from build123d import *

# Parameters (mm, degrees)
SKETCH2_W               = 100
SKETCH2_H               = 65
BOSS_EXTRUDE1_DEPTH     = 25
SKETCH3_W               = 40
SKETCH3_H               = 65
BOSS_EXTRUDE2_DEPTH     = 50
SKETCH4_W               = 50
SKETCH4_H               = 20
CUT_EXTRUDE1_DEPTH      = 40
CUT_EXTRUDE2_DEPTH      = 139.406105357
CUT_EXTRUDE2_DEPTH_BACK = 139.406105357
SKETCH5_W               = 41
SKETCH5_H               = 5.985076192
CUT_EXTRUDE4_START      = -25
SKETCH6_W               = 40
SKETCH6_H               = 25
CUT_EXTRUDE4_DEPTH      = 25


with BuildPart() as part:
    # Sketch2 → Boss-Extrude1 (new body)
    with BuildSketch(Plane(origin=(0, 0, 0), x_dir=(1, 0, 0), z_dir=(0, 1, 0))):
        Rectangle(SKETCH2_W, SKETCH2_H)
    extrude(amount=BOSS_EXTRUDE1_DEPTH)

    # Sketch3 → Boss-Extrude2 (add, symmetric)
    with BuildSketch(Plane(origin=(0, 0, 0), x_dir=(0, 0, -1), z_dir=(1, 0, 0))):
        with Locations((12.5, 57.5)):
            Rectangle(SKETCH3_W, SKETCH3_H)
    extrude(amount=BOSS_EXTRUDE2_DEPTH, both=True)

    # Sketch4 → Cut-Extrude1 (cut)
    with BuildSketch(Plane(origin=(0, 90, 0), x_dir=(1, 0, 0), z_dir=(0, 1, 0))):
        with Locations((0, 2.5)):
            Rectangle(SKETCH4_W, SKETCH4_H)
    extrude(amount=-CUT_EXTRUDE1_DEPTH, mode=Mode.SUBTRACT)

    # Sketch5 → Cut-Extrude2 (cut, two sides: drawn at the far end of the back side and taken through both)
    with BuildSketch(Plane(origin=(50, 0, 0), x_dir=(0, 0, -1), z_dir=(1, 0, 0)).offset(-CUT_EXTRUDE2_DEPTH_BACK)):
        with Locations((0, 2.992538096)):
            Rectangle(SKETCH5_W, SKETCH5_H)
    extrude(amount=CUT_EXTRUDE2_DEPTH + CUT_EXTRUDE2_DEPTH_BACK, mode=Mode.SUBTRACT)

    # Sketch6 → Cut-Extrude4 (cut)
    with BuildSketch(Plane.XY.offset(32.5).offset(CUT_EXTRUDE4_START)):
        with Locations((0, 12.5)):
            Rectangle(SKETCH6_W, SKETCH6_H)
    extrude(amount=CUT_EXTRUDE4_DEPTH, mode=Mode.SUBTRACT)


solid = part.part
Input: part model. Units: mm. Frame: model coordinates. A direction names the side the tool comes from. Round coordinates to 2 decimals unless told otherwise and drop trailing zeros. Order: outer loops, then holes, each group sorted by start corner. A loop starts at its lowest first (then second) coordinate and runs counter-clockwise, first axis right, second up. Notation, with made-up numbers: (26.5, 73.5) - (43.5, 73.5) arc R30 ccw to (43.5, 95.5) - close; hole circle Ø5 at (45.5, 36.25). An arc over 180 degrees is marked (long way). Answer as a JSON object with one key per item and string values. Group by question number.
(1) Reachability of faces 5 (the face through (-35, 25, 20)), 6 (the face through (-1, 5.985, 0)), 7 (the face through (20, 12, 20)) from +Z, -Z, +X, -X, +Y, -Y: full face, straight path, thin tool, end or side. Return the list, or none.
(2) Cut plane C-C (x = 29). Return loops of the section in (y, z).
(3) Draft query along Z for faces 1 (the face through (1, 44, -32.5)), 2 (the face through (35, 3, 20.5)), 3 (the face through (-25, 70, -2)), 4 (the face through (0, 70, -12.5)). Return one class per face: released by +Z, released by -Z, zero draft, split by the parting line, or undercut.
(4) Cut plane B-B (y = 15.5). Return loops of the section in (x, z), then the cut area to 3 significant figures.
(5) Cut plane D-D (y = 31). Return loops of the section in (x, z).
(6) Cut plane A-A (z = 3). Return loops of the section in (x, y).
(7) Material intervals for probe 1 along X at (y, z) = (22, 28.5); probe 2 along X at (y, z) = (61, 6); probe 3 along Z at (x, y) = (-31.5, 46), sorted ascending. Write a range as from..to.
(8) Pin query (flat end, axial travel): P1, Ø20, axis at x = 27.5, z = 26, coming from the +Y side; P2, Ø5, axis at x = 25.5, z = 13.5, coming from the -Y side; P3, Ø6, axis at x = -5, z = 2.5, coming from the +Y side. Return the tip coordinate at first contact, or that it passes through.
Here are the results:
{
 "1": {"face 5": "+Z, +X, -X, +Y", "face 6": "+X, -X, -Y", "face 7": "+Z, +Y, -Y"},
 "2": {"outline": "(0, -32.5) - (90, -32.5) - (90, 7.5) - (25, 7.5) - (25, 32.5) - (0, 32.5) - (0, 20.5) - (5.99, 20.5) - (5.99, -20.5) - (0, -20.5) - close"},
 "3": {"face 1": "released by -Z", "face 2": "undercut", "face 3": "zero draft", "face 4": "released by +Z"},
 "4": {"outline": "(-50, -32.5) - (50, -32.5) - (50, 32.5) - (20, 32.5) - (20, 7.5) - (-20, 7.5) - (-20, 32.5) - (-50, 32.5) - close", "area": "5,500 mm^2"},
 "5": {"outline": "(-50, -32.5) - (50, -32.5) - (50, 7.5) - (-50, 7.5) - close"},
 "6": {"outline": "(-50, 5.99) - (50, 5.99) - (50, 90) - (25, 90) - (25, 50) - (-25, 50) - (-25, 90) - (-50, 90) - close"},
 "7": {"probe 1": "x = -50..-20, 20..50", "probe 2": "x = -50..-25, 25..50", "probe 3": "z = -32.5..7.5"},
 "8": {"P1": "stops at y = 25", "P2": "stops at y = 5.99", "P3": "stops at y = 50"}
}
